Read the model definition and answer for the solid it produces. Units are mm, in the model's axes. Give positions to 0.01 mm unless a question says otherwise; leave off trailing zeros. Order: outer loops, then holes, each group sorted by start corner. A loop starts at its lowest first (then second) coordinate and runs counter-clockwise, first axis right, second up. Notation, with made-up numbers: M 12,64 L 39,64 A22 ccw 39,88 Z; hole C 27.25,65.5 d4. An arc over 180 degrees is marked long. One line per item, written item: value. Start each with the question number.
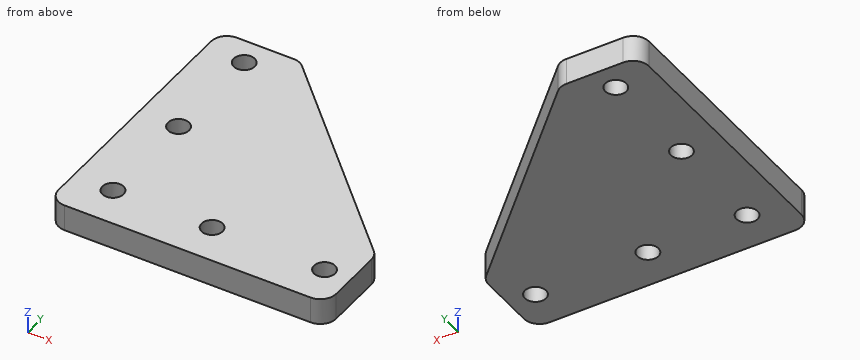
from build123d import *

# Parameters (mm, degrees)
SKETCH_1_R      = 2
EXTRUDE_1_DEPTH = 5
FILLET_1_R      = 3


with BuildPart() as part:
    # ｽｹｯﾁ1 → ﾎﾞｽ - 押し出し1 (new body)
    with BuildSketch(Plane.XY):
        Polygon((52.5, 15), (15, 52.5), (0, 52.5), (0, 0), (52.5, 0), align=None)
        with Locations((7.5, 7.5)):
            Circle(SKETCH_1_R, mode=Mode.SUBTRACT)
        with Locations((26.25, 7.5)):
            Circle(SKETCH_1_R, mode=Mode.SUBTRACT)
        with Locations((47.5, 7.5)):
            Circle(SKETCH_1_R, mode=Mode.SUBTRACT)
        with Locations((7.5, 27.5)):
            Circle(SKETCH_1_R, mode=Mode.SUBTRACT)
        with Locations((7.5, 47.5)):
            Circle(SKETCH_1_R, mode=Mode.SUBTRACT)
    extrude(amount=EXTRUDE_1_DEPTH)

    # ﾌｨﾚｯﾄ1
    fillet_1_edges = [part.edges().sort_by_distance(p)[0] for p in [
        (0, 0, 2.5),
        (0, 52.5, 2.5),
        (15, 52.5, 2.5),
        (52.5, 15, 2.5),
        (52.5, 0, 2.5),
    ]]
    fillet(fillet_1_edges, radius=FILLET_1_R)


solid = part.part
Q1. Find section B-B, the plane y = 7.5. Give the vertices of the cut face in (x, z).
Q2. This flat-tipped pin is pushed along its axis until it touches: pin 1 (6 mm diameter, centred on x = 35, y = 37, fed in from -Z). Where does it stop, or does it pass through?
Q3. Find section A-A, the plane x = 26.25. Give the vertices of the cut face in (y, z).
Q4. Find section C-C, the plane z = 1.85. Give the vertices of the cut face in (x, y).
Q5. Find section D-D, the plane y = 47.5. Give the vertices of the cut face in (x, z), then the cut area to 3 significant figures.
Q6. Consider probe 1 along Y at (x, z) = (7.5, 2.9); probe 2 along X at (y, z) = (9, 0.4); probe 3 along X at (y, z) = (8.5, 4.5). Determine where each line is inside the solid, lowest interval first.
Evaluation:
1. outline: M 0,0 L 5.5,0 L 5.5,5 L 0,5 Z; M 9.5,0 L 24.25,0 L 24.25,5 L 9.5,5 Z; M 28.25,0 L 45.5,0 L 45.5,5 L 28.25,5 Z; M 49.5,0 L 52.5,0 L 52.5,5 L 49.5,5 Z
2. pin 1: through
3. outline: M 0,0 L 5.5,0 L 5.5,5 L 0,5 Z; M 9.5,0 L 41.25,0 L 41.25,5 L 9.5,5 Z
4. outline: M 0,3 A3 ccw 3,0 L 49.5,0 A3 ccw 52.5,3 L 52.5,13.76 A3 ccw 51.62,15.88 L 15.88,51.62 A3 ccw 13.76,52.5 L 3,52.5 A3 ccw 0,49.5 Z; hole C 7.5,7.5 d4; hole C 7.5,27.5 d4; hole C 7.5,47.5 d4; hole C 26.25,7.5 d4; hole C 47.5,7.5 d4
5. outline: M 0,0 L 5.5,0 L 5.5,5 L 0,5 Z; M 9.5,0 L 20,0 L 20,5 L 9.5,5 Z
5. area: 80.0 mm2
6. probe 1: 0 to 5.5, 9.5 to 25.5, 29.5 to 45.5, 49.5 to 52.5
6. probe 2: 0 to 6.18, 8.82 to 24.93, 27.57 to 46.18, 48.82 to 52.5
6. probe 3: 0 to 5.77, 9.23 to 24.52, 27.98 to 45.77, 49.23 to 52.5
